from build123d import *

# Parameters (mm, degrees)
F1_DEPTH = 3.175
F2_D     = 1.778


with BuildPart() as f1:
    # F0 (on Top) → F1 (new body)
    with BuildSketch(Plane.XY):
        Polygon((-3.81, -5.08), (3.81, -5.08), (3.81, 0), (3.81, 2.54), (1.905, 5.08), (-3.81, 0), align=None)
        Polygon((1.905, 5.08), (3.81, 2.54), (3.81, 5.08), align=None)
    extrude(amount=F1_DEPTH)

    # F2 (through all)
    with Locations(Plane(origin=(0, 0, 0), x_dir=(1, 0, 0), z_dir=(0, 0, -1))):
        with Locations((2.8575, -3.81)):
            Hole(F2_D / 2)


solid = f1.part
Verification items for the finished model (mm, model axes). Give positions to 0.01 mm unless a question says otherwise; leave off trailing zeros. Loops run counter-clockwise (first coordinate to the right, second up) from the corner with the lowest first, then second, coordinate; pieces in that order, holes last.
1) Sectioned sample at C-C, the plane x = 3.25. Enter the section's corners in (y, z) (3 decimals), then the cut area to 3 significant figures.
2) Draft check along Y on faces 1 (the cylindrical face through (2.01, 3.54, 1.61)), 2 (the flat face through (3, 5.08, 2)), 3 (the flat face through (0, -1, 3.175)). Enter one of: pulls with the +Y half, pulls with the -Y half, needs draft (parallel to the pull), parting line crosses it, or undercut.
3) Depth check by flat-ended pin: pin 1 Ø1.1 at (x, y) = (2.86, 3.81) entering from +Z. Enter the tip coordinate at first touch or a pass-through.
4) Sectioned sample at B-B, the plane z = 1.3. Enter the section's corners in (x, y) (1 decimal), then the cut area to 3 significant figures.
5) Sectioned sample at D-D, the plane y = 2.5. Enter the section's corners in (x, z) (1 decimal).
6) Thickness scan on line 1 along Y through (x, z) = (3, 2.2); line 2 along Y through (x, z) = (1.25, 0.85); line 3 along Y through (x, z) = (2.25, 1.9). Record the ranges inside material, lowest first.
Answers:
1. outline: (-5.08, 0) - (3.012, 0) - (3.012, 3.175) - (-5.08, 3.175) - close; (4.608, 0) - (5.08, 0) - (5.08, 3.175) - (4.608, 3.175) - close
1. area: 27.2 mm2
2. face 1: undercut
2. face 2: pulls with the +Y half
2. face 3: needs draft
3. pin 1: passes through
4. outline: (-3.8, -5.1) - (3.8, -5.1) - (3.8, 5.1) - (1.9, 5.1) - (-3.8, 0) - close; hole circle Ø1.8 at (2.9, 3.8)
4. area: 60.4 mm2
5. outline: (-1, 0) - (3.8, 0) - (3.8, 3.2) - (-1, 3.2) - close
6. line 1: y = -5.08 to 2.93, 4.69 to 5.08
6. line 2: y = -5.08 to 4.5
6. line 3: y = -5.08 to 3.16, 4.46 to 5.08
